```python
from build123d import *

# Parameters (mm, degrees)
SKETCH002_R     = 5.45
SKETCH003_R     = 5
PAD001_DEPTH    = 10.25
SKETCH004_R     = 2.625
SKETCH004_R_2   = 1.11
POCKET_DEPTH    = 8
SKETCH005_R     = 3.43
SKETCH005_R_2   = 2.625
PAD002_DEPTH    = 1.95
FILLET_R        = 0.8
SKETCH_W        = 14.6
SKETCH_H        = 11.96
PAD_DEPTH       = 11.48
SKETCH006_W     = 10.03
SKETCH006_H     = 10.07
PAD003_DEPTH    = 5.75
POCKET001_DEPTH = 10.031
FILLET001_R     = 0.5
SKETCH008_R     = 1.815
POCKET002_DEPTH = 2
SKETCH009_W     = 4.14
SKETCH009_H     = 5.42
POCKET003_DEPTH = 0.67
CHAMFER_SIZE    = 0.65
SKETCH010_W     = 2.8
SKETCH010_H     = 2.07
POCKET004_DEPTH = 5


with BuildPart() as fillet_body:
    # Sketch001 → Loft section 0
    with BuildSketch(Plane.XY.offset(11.48)):
        with BuildLine():
            Line((-5.96, 5.42), (5.96, 5.42))
            ThreePointArc((6.46, 4.92), (6.313553, 5.273553), (5.96, 5.42))
            Line((6.46, 4.92), (6.46, -4.92))
            ThreePointArc((5.96, -5.42), (6.313553, -5.273553), (6.46, -4.92))
            Line((5.96, -5.42), (-5.96, -5.42))
            ThreePointArc((-6.46, -4.92), (-6.313553, -5.273553), (-5.96, -5.42))
            Line((-6.46, -4.92), (-6.46, 4.92))
            ThreePointArc((-5.96, 5.42), (-6.313553, 5.273553), (-6.46, 4.92))
        make_face()
    # Sketch002 → Loft section 1
    with BuildSketch(Plane.XY.offset(22.37)):
        Circle(SKETCH002_R)
    loft(ruled=True)

    # Sketch003 → Pad001 (new body)
    with BuildSketch(Plane.XY.offset(22.37)):
        Circle(SKETCH003_R)
    extrude(amount=PAD001_DEPTH)

    # Sketch004 → Pocket (cut)
    with BuildSketch(Plane.XY.offset(32.62)):
        Circle(SKETCH004_R)
        Circle(SKETCH004_R_2, mode=Mode.SUBTRACT)
    extrude(amount=-POCKET_DEPTH, mode=Mode.SUBTRACT)

    # Sketch005 → Pad002 (new body)
    with BuildSketch(Plane.XY.offset(32.62)):
        Circle(SKETCH005_R)
        Circle(SKETCH005_R_2, mode=Mode.SUBTRACT)
    extrude(amount=PAD002_DEPTH)

    # Fillet
    fillet_edges = [fillet_body.edges().sort_by_distance(p)[0] for p in [
        (-3.43, 0, 34.57),
    ]]
    fillet(fillet_edges, radius=FILLET_R)


with BuildPart() as fusion:
    # Sketch → Pad (new body)
    with BuildSketch(Plane.XY):
        Rectangle(SKETCH_W, SKETCH_H)
    extrude(amount=PAD_DEPTH)

    # Fusion: union Fillet body
    add(fillet_body.part)


with BuildPart() as obj1:
    # Sketch006 → Pad003 (new body)
    with BuildSketch(Plane(origin=(0, 0, 2.21), x_dir=(1, 0, 0), z_dir=(0, 0, -1))):
        with Locations((0, -2.335)):
            Rectangle(SKETCH006_W, SKETCH006_H)
    extrude(amount=PAD003_DEPTH)

    # Sketch007 → Pocket001 (cut, through all)
    with BuildSketch(Plane(origin=(-5.015, 0, 2.21), x_dir=(0, 1, 0), z_dir=(-1, 0, 0))):
        Polygon((15, 3.936222), (0, 6.460032), (0, 8.936222), (15, 8.936222), align=None)
    extrude(amount=-POCKET001_DEPTH, mode=Mode.SUBTRACT)

    # Fusion001: union Fusion
    add(fusion.part)

    # Fillet001
    fillet001_edges = [obj1.edges().sort_by_distance(p)[0] for p in [
        (7.3, 5.98, 5.74),
        (-7.3, 5.98, 5.74),
        (7.3, -5.98, 5.74),
        (-7.3, -5.98, 5.74),
    ]]
    fillet(fillet001_edges, radius=FILLET001_R)

    # Sketch008 → Pocket002 (cut)
    with BuildSketch(Plane(origin=(0, 7.37, 0), x_dir=(-1, 0, 0), z_dir=(0, 1, 0))):
        with Locations((-2.5075, -0.4)):
            Circle(SKETCH008_R)
        with Locations((2.5075, -0.4)):
            Circle(SKETCH008_R)
    extrude(amount=-POCKET002_DEPTH, mode=Mode.SUBTRACT)

    # Sketch009 → Pocket003 (cut)
    with BuildSketch(Plane(origin=(0, 0, -3.54), x_dir=(1, 0, 0), z_dir=(0, 0, -1))):
        with Locations((-2.535, -0.69)):
            Rectangle(SKETCH009_W, SKETCH009_H)
        with Locations((2.535, -0.69)):
            Rectangle(SKETCH009_W, SKETCH009_H)
    extrude(amount=-POCKET003_DEPTH, mode=Mode.SUBTRACT)

    # Chamfer
    chamfer_edges = [obj1.edges().sort_by_distance(p)[0] for p in [
        (2.535, 3.4, -3.54),
        (-2.535, 3.4, -3.54),
    ]]
    chamfer(chamfer_edges, length=CHAMFER_SIZE)

    # Sketch010 → Pocket004 (cut)
    with BuildSketch(Plane(origin=(0, 0, -2.87), x_dir=(1, 0, 0), z_dir=(0, 0, -1))):
        with Locations((-2.585, 0.655)):
            Rectangle(SKETCH010_W, SKETCH010_H)
        with Locations((2.585, 0.655)):
            Rectangle(SKETCH010_W, SKETCH010_H)
    extrude(amount=-POCKET004_DEPTH, mode=Mode.SUBTRACT)


solid = obj1.part
```
The listing builds one solid part. Answer for the finished solid, in the listing's coordinates (mm). A direction names the side the tool comes from. Coordinates: 2 decimals unless noted, no trailing zeros. Loops run counter-clockwise (first coordinate to the right, second up) from the corner with the lowest first, then second, coordinate; pieces in that order, holes last. Notation, with made-up numbers: M 32.25,24.25 L 46.25,24.25 A23 ccw 46.25,55.25 Z; hole C 4,34.5 d5. An arc over 180 degrees is marked long. Answer as CSV lines item,"result". Start each with the question number.
(1) The part is cut by section B-B (z = -0.4). Give the vertices of the cut face in (x, y) (1 decimal).
(2) The part is cut by section A-A (z = 4). Give the vertices of the cut face in (x, y), and give its area (3 significant figures).
(3) The mould has two halves that part along Y. Classify faces 1 (the flat face through (-1.185, -1, 0)), 2 (the flat face through (0, 0, -3.54)), 3 (the flat face through (0, -5.98, 6)): pulls with the +Y half, pulls with the -Y half, needs draft (parallel to the pull), parting line crosses it, or undercut.
(4) For faces 4 (the flat face through (-7.3, 0, 6)), 5 (the flat face through (0, -2.7, -2)), 6 (the flat face through (-3, -1.69, 0)), 7 (the cylindrical face through (-0.241, -1.084, 28.676)), determine the directions among +Z, -Z, +X, -X, +Y, -Y from which every point of the face is accessible in a straight line to the end or side of a thin tool.
(5) Given pin 1 (8 mm diameter, centred on x = 3.5, z = 14, fed in from +Y); pin 2 (1.8 mm diameter, centred on x = -2, z = 0, fed in from +Y); pin 3 (1 mm diameter, centred on y = -0.5, z = -1, fed in from +X) (3 decimals), each flat-ended and moving along its own axis, determine where each tip first touches the part or whether it passes through.
(6) Find the intervals of material crossed by L1, parallel to Y at x = 0, z = 28.5 (3 decimals); L2, parallel to Y at x = 0.25, z = 12; L3, parallel to Y at x = -1.5, z = 6.5, in increasing order. Write a range as [from, to].
Determined:
1,outline,"M -5,-2.7 L 5,-2.7 L 5,7.4 L 4.3,7.4 L 4.3,5.4 L 0.7,5.4 L 0.7,7.4 L -0.7,7.4 L -0.7,5.4 L -4.3,5.4 L -4.3,7.4 L -5,7.4 Z; hole M -4,-1.7 L -1.2,-1.7 L -1.2,0.4 L -4,0.4 Z; hole M 1.2,-1.7 L 4,-1.7 L 4,0.4 L 1.2,0.4 Z"
2,outline,"M -7.3,-5.48 A0.5 ccw -6.8,-5.98 L 6.8,-5.98 A0.5 ccw 7.3,-5.48 L 7.3,5.48 A0.5 ccw 6.8,5.98 L -6.8,5.98 A0.5 ccw -7.3,5.48 Z"
2,area,"174 mm2"
3,face 1,"undercut"
3,face 2,"needs draft"
3,face 3,"pulls with the -Y half"
4,face 4,"+Z, -Z, -X, +Y, -Y"
4,face 5,"-Z, +X, -X, -Y"
4,face 6,"-Z"
4,face 7,"+Z"
5,pin 1,"y = 5.98"
5,pin 2,"y = 5.37"
5,pin 3,"x = 5.015"
6,L1,"[-5, -2.625], [-1.11, 1.11], [2.625, 5]"
6,L2,"[-5.42, 5.42]"
6,L3,"[-5.98, 5.98]"
